from build123d import *

# Parameters (mm, degrees)
BOSS_EXTRUDE1_DEPTH = 3
CUT_EXTRUDE1_DEPTH  = 3


with BuildPart() as part:
    # Sketch4 → Boss-Extrude1 (new body)
    with BuildSketch(Plane.XY):
        with BuildLine():
            Line((0.18777702, -22.8), (-11.28722298, -22.8))
            Line((-11.28722298, -22.8), (-11.28722298, -14.972010466))
            ThreePointArc((-11.28722298, -14.972010466), (-0.162678986, 18.749294268), (11.545314563, -14.773903061))
            Line((11.545314563, -14.773903061), (11.66277702, -22.8))
            Line((11.66277702, -22.8), (0.18777702, -22.8))
        make_face()
    extrude(amount=BOSS_EXTRUDE1_DEPTH)

    # Sketch5 → Cut-Extrude1 (cut)
    with BuildSketch(Plane.XY):
        with BuildLine():
            Line((9.593685177, -14.576134767), (9.593685177, -20.570344852))
            Line((9.593685177, -20.570344852), (-9.514830363, -20.570344852))
            Line((-9.514830363, -20.570344852), (-9.514830363, -14.627730622))
            ThreePointArc((-9.514830363, -14.627730622), (-0.047117443, 17.449936388), (9.593685177, -14.576134767))
        make_face()
    extrude(amount=CUT_EXTRUDE1_DEPTH, mode=Mode.SUBTRACT)


solid = part.part
Geometry: final body of the model. Coordinates: model frame, mm. A direction names the side the tool comes from. Round coordinates to 2 decimals unless told otherwise and drop trailing zeros. Order: outer loops, then holes, each group sorted by start corner. A loop starts at its lowest first (then second) coordinate and runs counter-clockwise, first axis right, second up. Notation, with made-up numbers: (74, -33) -> (116, -33) arc R26 ccw to (116, -16) -> close; hole circle Ø7 at (40, 52). An arc over 180 degrees is marked (long way). Put each result on its own line as item: value. Start each with the question number.
Q1. Section C-C on z = 2.15. Return the cut outline in (x, y), and give its area (3 significant figures).
Q2. Line query: probe 1 along X at (y, z) = (0, 2.1); probe 2 along Y at (x, z) = (0, 2.05); probe 3 along Y at (x, z) = (15.5, 1.55). Output: solid intervals per line, ascending.
Q3. Section B-B on y = 0. Return the cut outline in (x, z).
Q4. Section A-A on x = 0. Return the cut outline in (y, z).
Q5. Pull-direction query (X, two-part tool) for faces 1 (the flat face through (11, -14, 3)), 2 (the cylindrical face through (-0.673, 17.437, 1.479)), 3 (the cylindrical face through (-0.815, 18.732, 1.479)); classes: +X half, -X half, draft (parallel to the pull), parting line (faces both ways), or undercut.
Q6. Reachability of faces 4 (the flat face through (11, -14, 0)), 5 (the flat face through (9.594, -18, 1)), 6 (the flat face through (-11.287, -19, 1)) from +Z, -Z, +X, -X, +Y, -Y: full face, straight path, thin tool, end or side. Return the list, or none.
Q7. First-contact query: pin 1 (1.5 mm diameter, centred on x = -4.5, z = 2, fed in from +Y); pin 2 (0.9 mm diameter, centred on y = -18.5, z = 1, fed in from -X); pin 3 (1 mm diameter, centred on x = 1.5, z = 2, fed in from +Y). Flat tips, straight axial feed; report the tip coordinate or a pass-through.
Ans:
1. outline: (-11.29, -22.8) -> (11.66, -22.8) -> (11.55, -14.77) arc R18.75 ccw (long way) to (-11.29, -14.97) -> close; hole (-9.51, -20.57) -> (9.59, -20.57) -> (9.59, -14.58) arc R17.45 ccw (long way) to (-9.51, -14.63) -> close
1. area: 192 mm2
2. probe 1: x = -18.75 to -17.45, 17.45 to 18.75
2. probe 2: y = -22.8 to -20.57, 17.45 to 18.75
2. probe 3: y = -10.55 to -8.02, 8.02 to 10.55
3. outline: (-18.75, 0) -> (-17.45, 0) -> (-17.45, 3) -> (-18.75, 3) -> close; (17.45, 0) -> (18.75, 0) -> (18.75, 3) -> (17.45, 3) -> close
4. outline: (-22.8, 0) -> (-20.57, 0) -> (-20.57, 3) -> (-22.8, 3) -> close; (17.45, 0) -> (18.75, 0) -> (18.75, 3) -> (17.45, 3) -> close
5. face 1: draft
5. face 2: undercut
5. face 3: parting line
6. face 4: -Z, +X, -X, +Y, -Y
6. face 5: +Z, -Z
6. face 6: +Z, -Z, -X, -Y
7. pin 1: stops at y = 18.37
7. pin 2: stops at x = -11.29
7. pin 3: stops at y = 18.72
